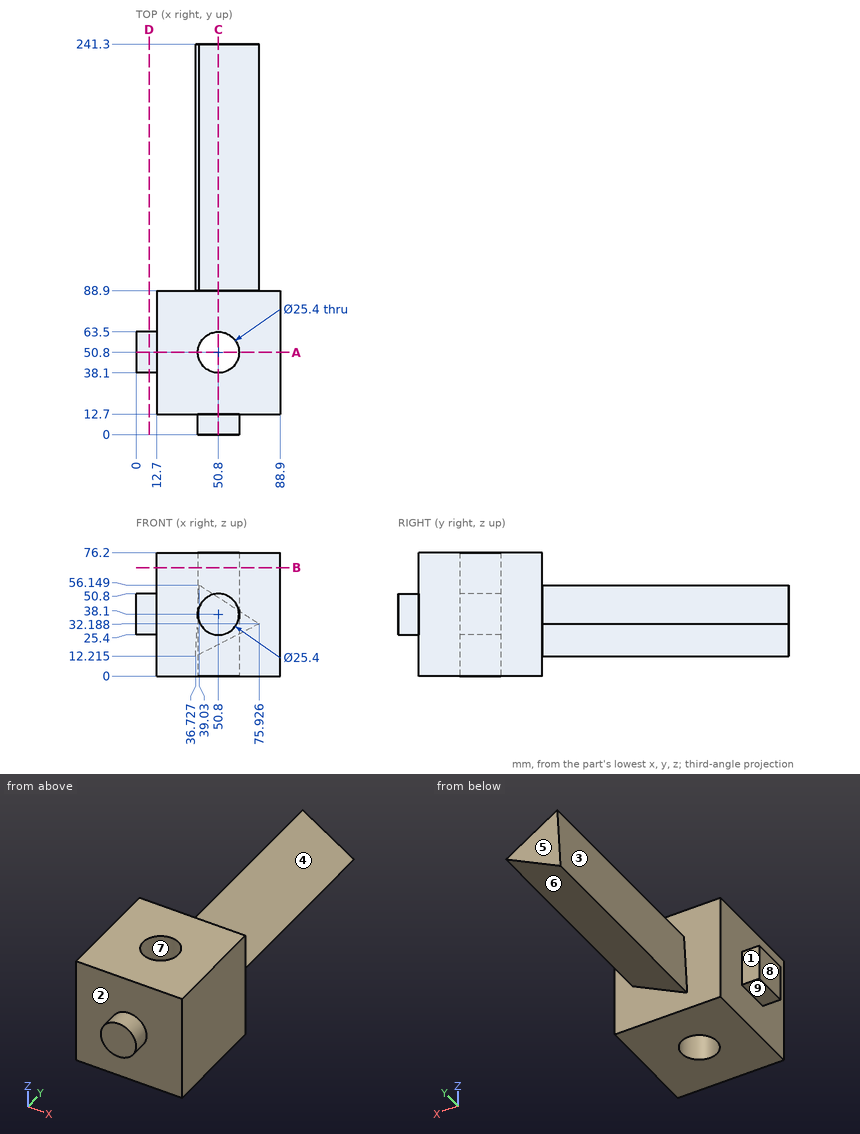
For this review, use the dimensioned drawing (mm, ordinates from the lowest corner) and the shaded views. A direction names the side the tool comes from. Coordinates: 2 decimals unless noted, no trailing zeros. Loops run counter-clockwise (first coordinate to the right, second up) from the corner with the lowest first, then second, coordinate; pieces in that order, holes last. Notation, with made-up numbers: (-19, 44.5) - (15, 44.5) arc R35 cw to (15, 83.5) - close; hole circle Ø8 at (34.25, 50.25). An arc over 180 degrees is marked (long way). Use one line per item in the form item = value. Start each with the question number.
1) Draft analysis for pull direction X (two halves, no side actions). For the marked faces 6, 7, 8 and 9, state which applies: released by +X, released by -X, zero draft, split by the parting line, or undercut.
2) Take a section at D-D (x = 8). State the section outline as (y, z) points, plus the area to 3 significant figures.
3) Take a section at A-A (y = 50.8). State the section outline as (x, z) points.
4) For pin 1 (5 mm diameter, centred on y = 75, z = 34, fed in from -X); pin 2 (10 mm diameter, centred on x = 4, y = 51, fed in from -Z); pin 3 (12 mm diameter, centred on x = 61.5, y = 148, fed in from +Z), all flat-tipped, find the tip position at first contact; note any pin that passes through.
5) Take a section at B-B (z = 67). State the section outline as (x, y) points, plus the area to 3 significant figures.
6) For the marked faces 1, 2, 3, 4 and 5, list the 3-axis set-ups (+Z, -Z, +X, -X, +Y, -Y) from which the entire face can be reached by the end or side of a thin tool; tool diameter is ignored.
7) To check wall thickness, follow probe 1 along X at (y, z) = (50, 30) (1 decimal); probe 2 along Y at (x, z) = (50, 27) (1 decimal); probe 3 along Y at (x, z) = (50, 24) (1 decimal). State the ranges of each line that lie inside material, in increasing order. Write a range as from..to.
8) Take a section at C-C (x = 50.8). State the section outline as (y, z) points (1 decimal).
From the geometry:
q1.face_6 = released by +X
q1.face_7 = undercut
q1.face_8 = released by -X
q1.face_9 = zero draft
q2.outline = (38.1, 25.4) - (63.5, 25.4) - (63.5, 50.8) - (38.1, 50.8) - close
q2.area = 645 mm2
q3.outline = (0, 25.4) - (12.7, 25.4) - (12.7, 0) - (38.1, 0) - (38.1, 76.2) - (12.7, 76.2) - (12.7, 50.8) - (0, 50.8) - close; (63.5, 0) - (88.9, 0) - (88.9, 76.2) - (63.5, 76.2) - close
q4.pin_1 = 12.7
q4.pin_2 = 25.4
q4.pin_3 = 45.45
q5.outline = (12.7, 12.7) - (88.9, 12.7) - (88.9, 88.9) - (12.7, 88.9) - close; hole circle Ø25.4 at (50.8, 50.8)
q5.area = 5,300 mm2
q6.face_1 = +Z, -Z, -X, +Y
q6.face_2 = -Y
q6.face_3 = +Z, -X, +Y
q6.face_4 = +Z, +X, +Y
q6.face_5 = +Z, -Z, +X, -X, +Y
q7.probe_1 = 0..38.1, 63.5..88.9
q7.probe_2 = 0..38.1, 63.5..241.3
q7.probe_3 = 12.7..38.1, 63.5..241.3
q8.outline = (0, 25.4) - (12.7, 25.4) - (12.7, 0) - (38.1, 0) - (38.1, 76.2) - (12.7, 76.2) - (12.7, 50.8) - (0, 50.8) - close; (63.5, 0) - (88.9, 0) - (88.9, 19.4) - (241.3, 19.4) - (241.3, 48.5) - (88.9, 48.5) - (88.9, 76.2) - (63.5, 76.2) - close
